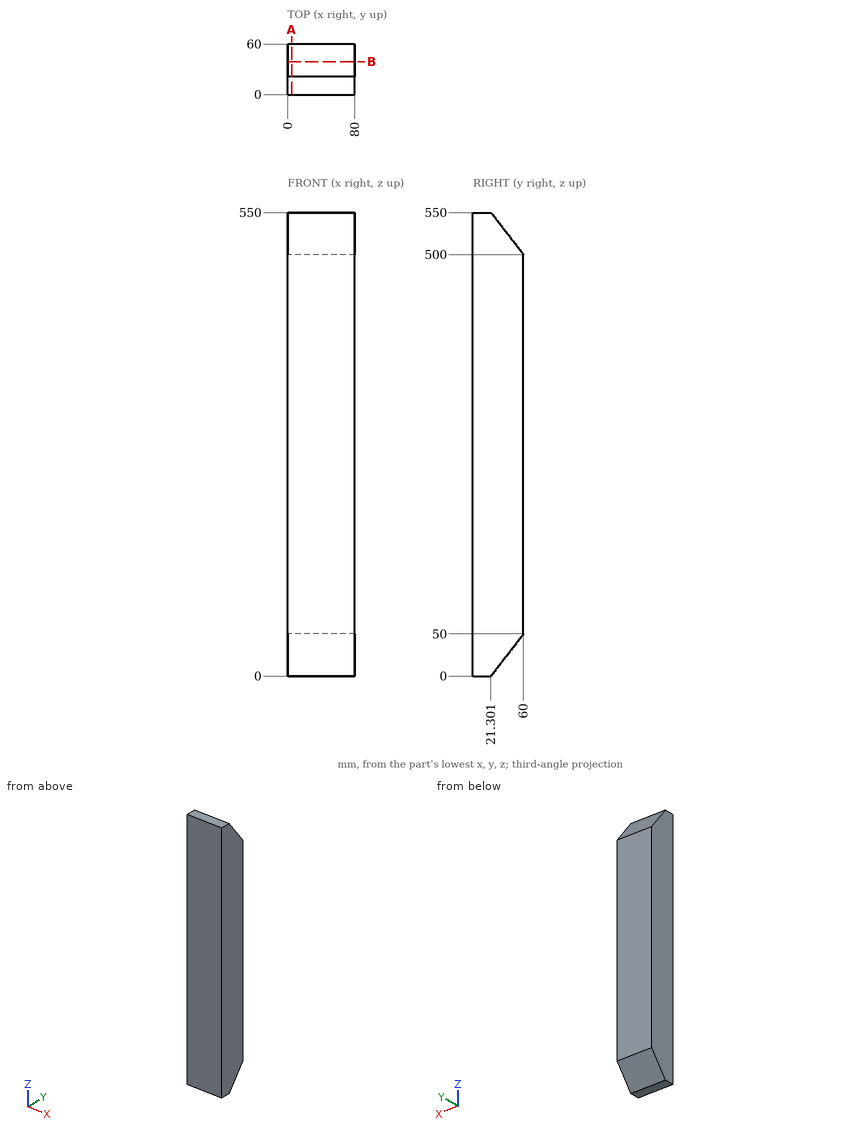
Input: dimensioned drawing with shaded views. Units: mm. Origin: part minimum x, y, z. Round coordinates to 2 decimals unless told otherwise and drop trailing zeros. Order: outer loops, then holes, each group sorted by start corner. A loop starts at its lowest first (then second) coordinate and runs counter-clockwise, first axis right, second up. Notation, with made-up numbers: (-37, 32.25) - (-14, 32.25) arc R12 ccw to (-14, 50.25) - close; hole circle Ø8 at (-31.5, 32). An arc over 180 degrees is marked (long way). Use CSV: the item, a comma, the result in double quotes. Start each with the question number.
Q1. Section query A-A (x = 5). Return loops of the section in (y, z).
Q2. Section query B-B (y = 39). Return loops of the section in (x, z).
Q3. First-contact query: pin 1 (4 mm diameter, centred on x = 38, y = 32.5, fed in from -Z) (1 decimal); pin 2 (12 mm diameter, centred on x = 31, y = 49, fed in from +Z) (1 decimal). Flat tips, straight axial feed; report the tip coordinate or a pass-through.
Q4. Material intervals for line 1 along Z through (x, y) = (35, 34.5) (1 decimal); line 2 along Y through (x, z) = (14, 522); line 3 along Y through (x, z) = (27.5, 516.5), sorted ascending. Write a range as from..to.
Result set:
1,outline,"(0, 0) - (21.3, 0) - (60, 50) - (60, 500) - (21.3, 550) - (0, 550) - close"
2,outline,"(0, 22.87) - (80, 22.87) - (80, 527.13) - (0, 527.13) - close"
3,pin 1,"stops at z = 11.9"
3,pin 2,"stops at z = 522"
4,line 1,"z = 17.1..532.9"
4,line 2,"y = 0..42.97"
4,line 3,"y = 0..47.23"
